Autodesk Inventor part; units mm, degrees
ref_plane "YZ Plane" through (0, 0, 0) normal (1, 0, 0) x (0, 1, 0)
ref_plane "XZ Plane" through (0, 0, 0) normal (0, 1, 0) x (-1, 0, 0)
ref_plane "XY Plane" through (0, 0, 0) normal (0, 0, 1) x (1, 0, 0)
ref_plane "Work Plane1" through (0, 0, 0) normal (0, 0, 1) x (1, 0, 0)
sketch "Sketch1" plane through (0, 0, 0) normal (0, 0, 1) x (1, 0, 0)
  line L0 (0, 0) -> (304.8, 0)
  line L1 (304.8, 0) -> (292.1, 0)
  line L2 (-330.2, 20) -> (330.2, 20)
  line L3 (-330.2, 0) -> (-330.2, 20)
  line L4 (330.2, 0) -> (-330.2, 0)
  line L5 (330.2, 20) -> (330.2, 0)
  line L6 (292.1, 0) -> (292.1, 10)
  line L7 (330.6445, 0) -> (253.5555, 0)
  line L8 (253.5555, 0) -> (253.5555, 20)
  line L9 (253.5555, 20) -> (330.6445, 20)
  line L10 (330.6445, 20) -> (330.6445, 0)
  line L11 (330.6445, 0) -> (253.5555, 20) construction
  line L12 (253.5555, 0) -> (330.6445, 20) construction
  line L13 (330.6445, 0) -> (330.6445, -76.2)
  line L14 (330.6445, 0) -> (406.8445, 0) construction
  line L15 (330.6445, -76.2) -> (310.8751, -76.2)
  line L16 (330.6445, 20) -> (229.0445, 20)
  line L17 (229.0445, 20) -> (229.0445, 0)
  line L18 (229.0445, 0) -> (310.8751, -76.2)
  line L19 (310.8751, -76.2) -> (310.8751, 0)
  dimension "d0" = 304.8
  dimension "d1" = 12.7
  dimension "d2" = 76.2
  dimension "d3" = 90
  dimension "d4" = 101.6
extrude "Extrusion1" add sketch "Sketch1" along normal blind 5.08 contours L17 L2 L8 L0 | L0 L4 L19 L18 | L8 L2 L5 L4 L0 | L19 L4 L7 L13 L15 | L9 L10 L7 L5
sketch "Sketch2" plane through (0, 0, 5.08) normal (0, 0, 1) x (1, 0, 0)
  line L0 (310.2, -876.3) -> (310.2, 0)
  line L1 (310.2, 0) -> (297.5, 0)
  line L2 (297.5, 0) -> (297.5, 10)
  line L3 (284.8, 20) -> (310.2, 20)
  line L4 (310.2, 20) -> (310.2, 0)
  line L5 (310.2, 0) -> (284.8, 0)
  line L6 (284.8, 0) -> (284.8, 20)
  line L7 (284.8, 20) -> (310.2, 0) construction
  line L8 (310.2, 20) -> (284.8, 0) construction
  point P0 (0, 0)
  dimension "d7" = 12.7
  dimension "d8" = 10
  dimension "d9" = 90
extrude "Extrusion2" add sketch "Sketch2" along normal blind 25.4
sketch "Sketch3" plane through (229.0445, 20, 0) normal (0, 1, 0) x (1, 0, 0)
  line L0 (101.6, 0) -> (0, 0)
  line L1 (0, 0) -> (0, -5.08)
  line L2 (55.7555, -5.08) -> (0, -5.08)
  line L3 (55.7555, -5.08) -> (55.7555, -30.48)
  line L4 (81.1555, -30.48) -> (55.7555, -30.48)
  line L5 (81.1555, -5.08) -> (81.1555, -30.48)
  line L6 (101.6, -5.08) -> (81.1555, -5.08)
  line L7 (101.6, 0) -> (101.6, -5.08)
  circle A0 centre (68.4555, -22.86) radius 4
  point P0 (-229.0445, 0)
  dimension "d12" = 8
  dimension "d13" = 7.62
extrude "Extrusion3" cut sketch "Sketch3" against normal blind 101.6 contours A0
chamfer "Chamfer1" distance 14.2875 angle 45 2 edges at (284.8, 10, 5.08) (310.2, 10, 5.08)
sketch "Sketch4" plane through (0, 0, 5.08) normal (0, 0, 1) x (1, 0, 0)
  line L0 (324.4875, 0) -> (324.4875, 20)
  line L1 (324.4875, 0) -> (270.5125, 0)
  line L2 (270.5125, 20) -> (270.5125, 0)
  line L3 (270.5125, 20) -> (229.0445, 20)
  line L4 (229.0445, 20) -> (229.0445, 0)
  line L5 (229.0445, 0) -> (310.8751, -76.2)
  line L6 (310.8751, -76.2) -> (330.6445, -76.2)
  line L7 (330.6445, -76.2) -> (330.6445, 20)
  line L8 (330.6445, 20) -> (324.4875, 20)
  line L9 (330.2, 0) -> (330.2, -876.3)
  line L10 (310.2, 0) -> (330.2, 0)
  line L11 (310.2, -876.3) -> (310.2, 0)
  line L12 (330.2, -876.3) -> (310.2, -876.3)
  line L13 (324.4875, 0) -> (324.4875, 20)
  line L14 (324.4875, 0) -> (270.5125, 0)
  line L15 (270.5125, 20) -> (270.5125, 0)
  line L16 (270.5125, 20) -> (229.0445, 20)
  line L17 (229.0445, 20) -> (229.0445, 0)
  line L18 (229.0445, 0) -> (310.8751, -76.2)
  line L19 (310.8751, -76.2) -> (330.6445, -76.2)
  line L20 (330.6445, -76.2) -> (330.6445, 20)
  line L21 (330.6445, 20) -> (324.4875, 20)
  line L22 (330.2, 0) -> (-330.2, 0)
  circle A0 centre (320.7598, -50.8) radius 2.5
  circle A1 centre (320.7598, -19.05) radius 2.5
  circle A2 centre (241.7445, 10) radius 2.5
  circle A3 centre (260.7945, 10) radius 2.5
  point P0 (0, 0)
  dimension "d19" = 5
  dimension "d20" = 5
  dimension "d21" = 31.75
  dimension "d22" = 25.4
  dimension "d23" = 5
  dimension "d24" = 5
  dimension "d25" = 12.7
  dimension "d26" = 19.05
extrude "Extrusion4" cut sketch "Sketch4" against normal blind 101.6 contours A0 | A1 | A2 | A3
properties part number "Bed Bracket"
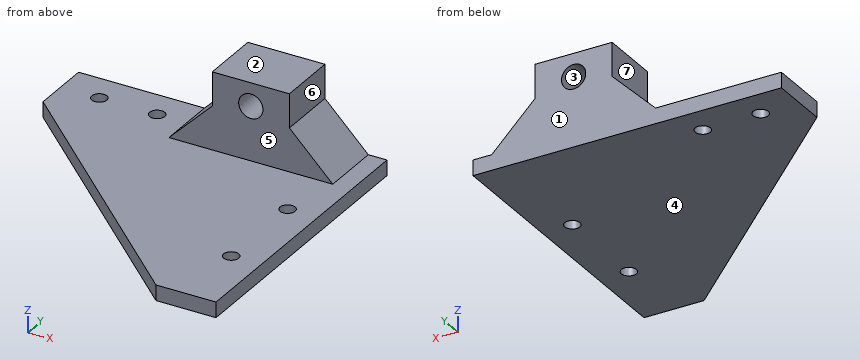
Model file for the job. Use its own axes, mm. Face numbers are marked on the shaded views. A direction names the side the tool comes from. Coordinates: 2 decimals unless noted, no trailing zeros. Loops run counter-clockwise (first coordinate to the right, second up) from the corner with the lowest first, then second, coordinate; pieces in that order, holes last. Notation, with made-up numbers: (-21.5, 55) - (19.5, 55) arc R19 ccw to (19.5, 80) - close; hole circle Ø8 at (76.5, 51). An arc over 180 degrees is marked (long way). Answer as a JSON object with one key per item and string values. Group by question number.
(1) Cut at A-A (z = 22.86). Give the cut face in (x, y).
(2) Tool access for the marked faces 5, 6 and 7: list every direction of +Z, -Z, +X, -X, +Y, -Y with a clear straight run to the whole face (end or side of a thin tool).
(3) Flat gauge pins, fed straight in: pin 1 (6 mm diameter, centred on x = 320.76, y = -50.8, fed in from +Z); pin 2 (7 mm diameter, centred on x = 297.5, z = 22.86, fed in from +Y); pin 3 (5.5 mm diameter, centred on y = 8, z = 26.5, fed in from -X); pin 4 (4 mm diameter, centred on x = 302.5, z = 21, fed in from -Y). Where does each tip first touch, or does it go through?
(4) Probe line 1 along Z through (x, y) = (319, -41); line 2 along Z through (x, y) = (295, 6.5); line 3 along Y through (x, z) = (310, 28). List the from-to ranges inside material, lowest first.
(5) Cut at C-C (x = 296). Give the cut face in (y, z).
(6) Two-plate mould, pull along Z, no slides. Class the marked faces 1, 2, 3 and 4: released by +Z, released by -Z, zero draft, split by the parting line, or undercut.
(7) Cut at D-D (y = -19.05). Give the cut face in (x, z), then the cut area to 3 significant figures.
(8) Cut at B-B (y = 10). Give the cut face in (x, z), then the cut area to 3 significant figures.
Geometry says:
{
 "1": {"outline": "(284.8, 0) - (293.5, 0) - (293.5, 20) - (284.8, 20) - close; (301.5, 0) - (310.2, 0) - (310.2, 20) - (301.5, 20) - close"},
 "2": {"face 5": "+Z, +X, -X, -Y", "face 6": "+Z, +X, +Y, -Y", "face 7": "+Z, -X, +Y, -Y"},
 "3": {"pin 1": "stops at z = 5.08", "pin 2": "passes through", "pin 3": "stops at x = 284.8", "pin 4": "stops at y = 0"},
 "4": {"line 1": "z = 0 to 5.08", "line 2": "z = 0 to 19.74, 25.98 to 30.48", "line 3": "y = 0 to 20"},
 "5": {"outline": "(-62.35, 0) - (20, 0) - (20, 19.15) - (0, 19.15) - (0, 5.08) - (-62.35, 5.08) - close; (0, 26.57) - (20, 26.57) - (20, 30.48) - (0, 30.48) - close"},
 "6": {"face 1": "zero draft", "face 2": "released by +Z", "face 3": "undercut", "face 4": "released by -Z"},
 "7": {"outline": "(249.5, 0) - (318.26, 0) - (318.26, 5.08) - (249.5, 5.08) - close; (323.26, 0) - (330.64, 0) - (330.64, 5.08) - (323.26, 5.08) - close", "area": "387 mm^2"},
 "8": {"outline": "(229.04, 0) - (239.24, 0) - (239.24, 5.08) - (229.04, 5.08) - close; (244.24, 0) - (258.29, 0) - (258.29, 5.08) - (244.24, 5.08) - close; (263.29, 0) - (330.64, 0) - (330.64, 5.08) - (324.49, 5.08) - (310.2, 19.37) - (310.2, 30.48) - (284.8, 30.48) - (284.8, 19.37) - (270.51, 5.08) - (263.29, 5.08) - close; hole circle Ø8 at (297.5, 22.86)", "area": "1,260 mm^2"}
}
